from build123d import *

# Parameters (mm, degrees)
F0_R      = 53.34
F0_R_2    = 22.225
F1_DEPTH  = 304.8
F4_R      = 53.34
F4_R_2    = 30.48
F5_DEPTH  = 101.6
F10_R     = 12.7
F10_R_2   = 8.89
F10_R_3   = 3.175
F11_DEPTH = 15.24
F12_DEPTH = 27.94
F13_DEPTH = 32.3429548439
F14_R     = 12.7
F14_R_2   = 8.89
F14_R_3   = 3.175
F15_DEPTH = 15.24
F16_DEPTH = 27.94
F17_DEPTH = 32.3429548439
F18_R     = 12.7
F19_DEPTH = 15.24
F20_R     = 12.7
F21_DEPTH = 15.24


with BuildPart() as f1:
    # F0 (on Front) → F1 (new body, symmetric)
    with BuildSketch(Plane.XZ):
        Circle(F0_R)
        Circle(F0_R_2, mode=Mode.SUBTRACT)
    extrude(amount=F1_DEPTH, both=True)

    # F4 (on offset) → F5 (cut)
    with BuildSketch(Plane(origin=(0, 304.8, 0), x_dir=(-1, 0, 0), z_dir=(0, 1, 0))):
        Circle(F4_R)
        Circle(F4_R_2, mode=Mode.SUBTRACT)
    extrude(amount=-F5_DEPTH, mode=Mode.SUBTRACT)

    # F6 (on Right) → F7 (revolve)
    with BuildSketch(Plane.YZ):
        Polygon((203.2, 53.34), (203.2, 30.48), (226.06, 30.48), align=None)
    revolve(axis=Axis((0, 101.6, 0), (0, 1, 0)))

    # F10 (on offset) → F11 (cut)
    with BuildSketch(Plane.XY.offset(53.34)):
        Circle(F10_R)
        Circle(F10_R_2, mode=Mode.SUBTRACT)
        Circle(F10_R_2)
        Circle(F10_R_3, mode=Mode.SUBTRACT)
        Circle(F10_R_3)
    extrude(amount=-F11_DEPTH, mode=Mode.SUBTRACT)

    # F10 (on offset) → F12 (cut)
    with BuildSketch(Plane.XY.offset(53.34)):
        Circle(F10_R_2)
        Circle(F10_R_3, mode=Mode.SUBTRACT)
        Circle(F10_R_3)
    extrude(amount=-F12_DEPTH, mode=Mode.SUBTRACT)

    # F10 (on offset) → F13 (cut, up to face)
    with BuildSketch(Plane.XY.offset(53.34)):
        Circle(F10_R_3)
    extrude(amount=-F13_DEPTH, mode=Mode.SUBTRACT)

    # F14 (on offset) → F15 (cut)
    with BuildSketch(Plane.XY.offset(-53.34)):
        Circle(F14_R)
        Circle(F14_R_2, mode=Mode.SUBTRACT)
        Circle(F14_R_2)
        Circle(F14_R_3, mode=Mode.SUBTRACT)
        Circle(F14_R_3)
    extrude(amount=F15_DEPTH, mode=Mode.SUBTRACT)

    # F14 (on offset) → F16 (cut)
    with BuildSketch(Plane.XY.offset(-53.34)):
        Circle(F14_R_2)
        Circle(F14_R_3, mode=Mode.SUBTRACT)
        Circle(F14_R_3)
    extrude(amount=F16_DEPTH, mode=Mode.SUBTRACT)

    # F14 (on offset) → F17 (cut, up to face)
    with BuildSketch(Plane.XY.offset(-53.34)):
        Circle(F14_R_3)
    extrude(amount=F17_DEPTH, mode=Mode.SUBTRACT)

    # F18 (on offset) → F19 (join, through all)
    with BuildSketch(Plane.XY.offset(53.34)):
        Circle(F18_R)
    extrude(amount=-F19_DEPTH)

    # F20 (on offset) → F21 (join, through all)
    with BuildSketch(Plane.XY.offset(-53.34)):
        Circle(F20_R)
    extrude(amount=F21_DEPTH)


solid = f1.part
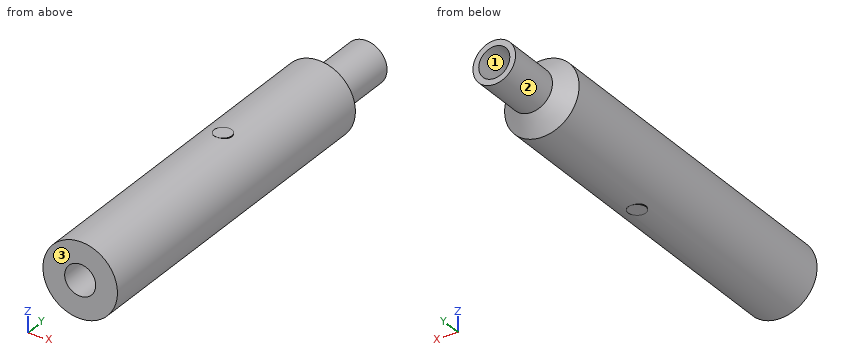
The listing builds one solid part. Answer for the finished solid, in the listing's coordinates (mm). Face numbers are marked on the shaded views. Coordinates: 2 decimals unless noted, no trailing zeros. Order: outer loops, then holes, each group sorted by start corner. A loop starts at its lowest first (then second) coordinate and runs counter-clockwise, first axis right, second up. Notation, with made-up numbers: (89.25, 33.25) -> (121.25, 33.25) arc R33 ccw to (121.25, 64.25) -> close; hole circle Ø10 at (86, 19.25). An arc over 180 degrees is marked (long way). Answer in a Markdown table with one row per item. Add a question column.
Item 1: Find section B-B (y = 93). Write down the section's boundary in (x, z) (3 decimals), then the cut area to 3 significant figures.
Item 2: Each of these flat-tipped pins is pushed along its axis until it touches: P1, Ø1.5, axis at y = 138, z = 2.5, coming from the +X side; P2, Ø1, axis at x = -8.5, y = -65, coming from the +Z side; P3, Ø6, axis at y = 181.5, z = 28, coming from the +X side. Where does it stop, or does it pass through?
Item 3: Find the intervals of material crossed by L1, parallel to Y at x = 0, z = 29; L2, parallel to X at y = 97.5, z = -3.5; L3, parallel to Z at x = 0, y = 27.5 (3 decimals), in increasing order. Write a range as from..to.
Item 4: Find section A-A (z = 0). Write down the section's boundary in (x, y) (3 decimals), then the cut area to 3 significant figures.
Item 5: Determine the mould class of the marked faces 1, 2 and 3 for opening direction Z: +Z half, -Z half, draft (parallel to the pull), parting line (faces both ways), or undercut.
Result set:
| question | item | result |
|---|---|---|
| 1 | outline | circle Ø106.68 at (0, 0); hole circle Ø44.45 at (0, 0) |
| 1 | area | 7,390 mm² |
| 2 | P1 | stops at x = 53.31 |
| 2 | P2 | stops at z = 52.74 |
| 2 | P3 | stops at x = 47.12 |
| 3 | L1 | y = -304.8..-8.89, 8.89..304.8 |
| 3 | L2 | x = -53.23..-21.95, 21.95..53.23 |
| 3 | L3 | z = -53.34..-22.225, 22.225..53.34 |
| 4 | outline | (-53.34, -304.8) -> (-22.225, -304.8) -> (-22.225, 304.8) -> (-30.48, 304.8) -> (-30.48, 226.06) -> (-53.34, 203.2) -> close; (22.225, -304.8) -> (53.34, -304.8) -> (53.34, 203.2) -> (30.48, 226.06) -> (30.48, 304.8) -> (22.225, 304.8) -> close |
| 4 | area | 33,800 mm² |
| 5 | face 1 | undercut |
| 5 | face 2 | parting line |
| 5 | face 3 | draft |
